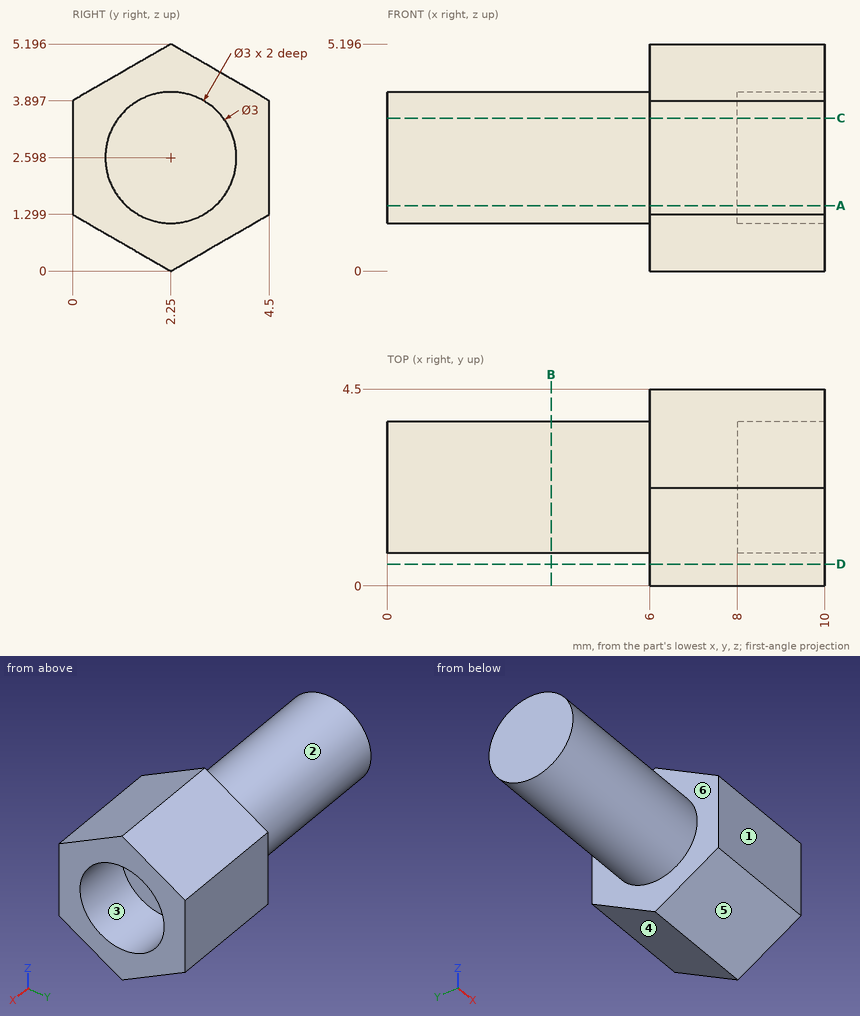
Part print with two shaded views. Sizes in mm from the minimum x, y, z corner. A direction names the side the tool comes from. Round coordinates to 2 decimals unless told otherwise and drop trailing zeros. Loops run counter-clockwise (first coordinate to the right, second up) from the corner with the lowest first, then second, coordinate; pieces in that order, holes last. Notation, with made-up numbers: M -34.5,40.5 L -16.5,40.5 A15 ccw -16.5,59.5 Z; hole C 11,-17 d8. An arc over 180 degrees is marked long. Put each result on its own line as item: value. Start each with the question number.
Item 1: Drop flat-ended pins along their axis: P1, Ø2.5, axis at y = 2.25, z = 2.6, coming from the +X side; P2, Ø3, axis at x = 3, z = 1, coming from the +Y side; P3, Ø2, axis at x = 2, y = 1, coming from the +Z side. Give the stop position or say it passes through.
Item 2: 3-axis set-ups, long thin cutter, end or side, ignore diameter. For the marked faces 5 and 6: which of +Z, -Z, +X, -X, +Y, -Y reach the whole face in a straight line?
Item 3: Cut at A-A (z = 1.5). List the corners of the cut face in (x, y).
Item 4: Cut at B-B (x = 3.75). List the corners of the cut face in (y, z).
Item 5: Cut at C-C (z = 3.5). List the corners of the cut face in (x, y), then the cut area to 3 significant figures.
Item 6: Drill centre lines: line 1 along X through (y, z) = (3.3, 2.25); line 2 along X through (y, z) = (3.55, 0.85); line 3 along Z through (x, y) = (9, 1.05). Where is each one in solid material? Low to high.
Item 7: Cut at D-D (y = 0.5). List the corners of the cut face in (x, z), then the cut area to 3 significant figures.
Item 8: Mould opens along Y. For the marked faces 1, 2, 3 and 4 say: released by +Y, released by -Y, zero draft, split by the parting line, or undercut.
Answer block:
1. P1: x = 8
1. P2: y = 3.75
1. P3: z = 4.08
2. face 5: -Z, +X, -X, -Y
2. face 6: -X
3. outline: M 0,1.23 L 6,1.23 L 6,0 L 10,0 L 10,1.23 L 8,1.23 L 8,3.27 L 10,3.27 L 10,4.5 L 6,4.5 L 6,3.27 L 0,3.27 Z
4. outline: C 2.25,2.6 d3
5. outline: M 0,1.05 L 6,1.05 L 6,0 L 10,0 L 10,1.05 L 8,1.05 L 8,3.45 L 10,3.45 L 10,4.5 L 6,4.5 L 6,3.45 L 0,3.45 Z
5. area: 27.6 mm2
6. line 1: 0 to 8
6. line 2: 6 to 10
6. line 3: 0.69 to 1.7, 3.5 to 4.5
7. outline: M 6,1.01 L 10,1.01 L 10,4.19 L 6,4.19 Z
7. area: 12.7 mm2
8. face 1: released by -Y
8. face 2: split by the parting line
8. face 3: undercut
8. face 4: released by +Y
